from build123d import *

# Parameters (mm, degrees)
F0_R     = 3.7465
F1_DEPTH = 29.718
F2_W     = 1.5875
F2_H     = 6.35
F3_DEPTH = 10.16
F4_R     = 1.5875
F5_DEPTH = 25.4


with BuildPart() as f1:
    # F0 (on Top) → F1 (new body)
    with BuildSketch(Plane.XY):
        Circle(F0_R)
    extrude(amount=F1_DEPTH)

    # F2 (on Right) → F3 (join, symmetric)
    with BuildSketch(Plane.YZ):
        with Locations((-0.79375, 3.175)):
            Rectangle(F2_W, F2_H)
        with Locations((0.79375, 3.175)):
            Rectangle(F2_W, F2_H)
    extrude(amount=F3_DEPTH, both=True)

    # F4 (on face) → F5 (cut)
    with BuildSketch(Plane.YZ.offset(10.16)):
        with Locations((0, 23.368)):
            Circle(F4_R)
    extrude(amount=-F5_DEPTH, mode=Mode.SUBTRACT)


solid = f1.part
Model file for the job. Use its own axes, mm. A direction names the side the tool comes from. Give positions to 0.01 mm unless a question says otherwise; leave off trailing zeros. Loops run counter-clockwise (first coordinate to the right, second up) from the corner with the lowest first, then second, coordinate; pieces in that order, holes last.
1) Flat gauge pins, fed straight in: pin 1 Ø2 at (y, z) = (2.5, 12.5) entering from +X; pin 2 Ø1 at (x, z) = (-6, 10.5) entering from -Y; pin 3 Ø1 at (x, y) = (6, -0.5) entering from +Z; pin 4 Ø1.9 at (x, z) = (7.5, 4) entering from +Y. Where does each tip first touch, or does it go through?
2) Pull direction Y, two halves, no side cores. Call faces 5 (the flat face through (7, -1.588, 3)), 6 (the cylindrical face through (0.051, -0.344, 21.818)), 7 (the flat face through (-7, 1.588, 3)): +Y half, -Y half, draft (parallel to the pull), parting line (faces both ways), or undercut.
3) Tool access for faces 1 (the flat face through (7, 1.588, 3)), 2 (the flat face through (-7, -1.588, 3)), 3 (the flat face through (10.16, 0, 3)), 4 (the cylindrical face through (-3.743, 0.165, 14.651)): list every direction of +Z, -Z, +X, -X, +Y, -Y with a clear straight run to the whole face (end or side of a thin tool).
4) Saw through at B-B (z = 4). Write the cut outline in (x, y), plus the area to 3 significant figures.
5) Saw through at A-A (y = 0). Write the cut outline in (x, z), plus the area to 3 significant figures.
6) Saw through at C-C (x = 2.25). Write the cut outline in (y, z) (1 decimal), plus the area to 3 significant figures.
7) Saw through at D-D (z = 22.5). Write the cut outline in (x, y), plus the area to 3 significant figures.
8) Wall check: line 1 (Z direction, x = 0.75, y = 0); line 2 (Z direction, x = 8, y = 1.5); line 3 (X direction, y = 0, z = 21.25). Give the ranges that are in metal, low to high.
Answer block:
1. pin 1: stops at x = 3.43
1. pin 2: passes through
1. pin 3: stops at z = 6.35
1. pin 4: stops at y = 1.59
2. face 5: -Y half
2. face 6: undercut
2. face 7: +Y half
3. face 1: +Z, -Z, +X, +Y
3. face 2: +Z, -Z, -X, -Y
3. face 3: +Z, -Z, +X, +Y, -Y
3. face 4: +Z
4. outline: (-10.16, -1.59) - (-3.39, -1.59) arc R3.75 ccw to (3.39, -1.59) - (10.16, -1.59) - (10.16, 1.59) - (3.39, 1.59) arc R3.75 ccw to (-3.39, 1.59) - (-10.16, 1.59) - close
4. area: 85.6 mm2
5. outline: (-10.16, 0) - (10.16, 0) - (10.16, 6.35) - (3.75, 6.35) - (3.75, 21.78) - (-3.75, 21.78) - (-3.75, 6.35) - (-10.16, 6.35) - close; (-3.75, 24.96) - (3.75, 24.96) - (3.75, 29.72) - (-3.75, 29.72) - close
5. area: 280 mm2
6. outline: (-3, 0) - (3, 0) - (3, 29.7) - (-3, 29.7) - close; hole circle Ø3.2 at (0, 23.4)
6. area: 170 mm2
7. outline: (-3.5, -1.33) arc R3.75 ccw to (3.5, -1.33) - close; (-3.5, 1.33) - (3.5, 1.33) arc R3.75 ccw to start
7. area: 24.6 mm2
8. line 1: z = 0 to 21.78, 24.96 to 29.72
8. line 2: z = 0 to 6.35
8. line 3: x = -3.75 to 3.75
